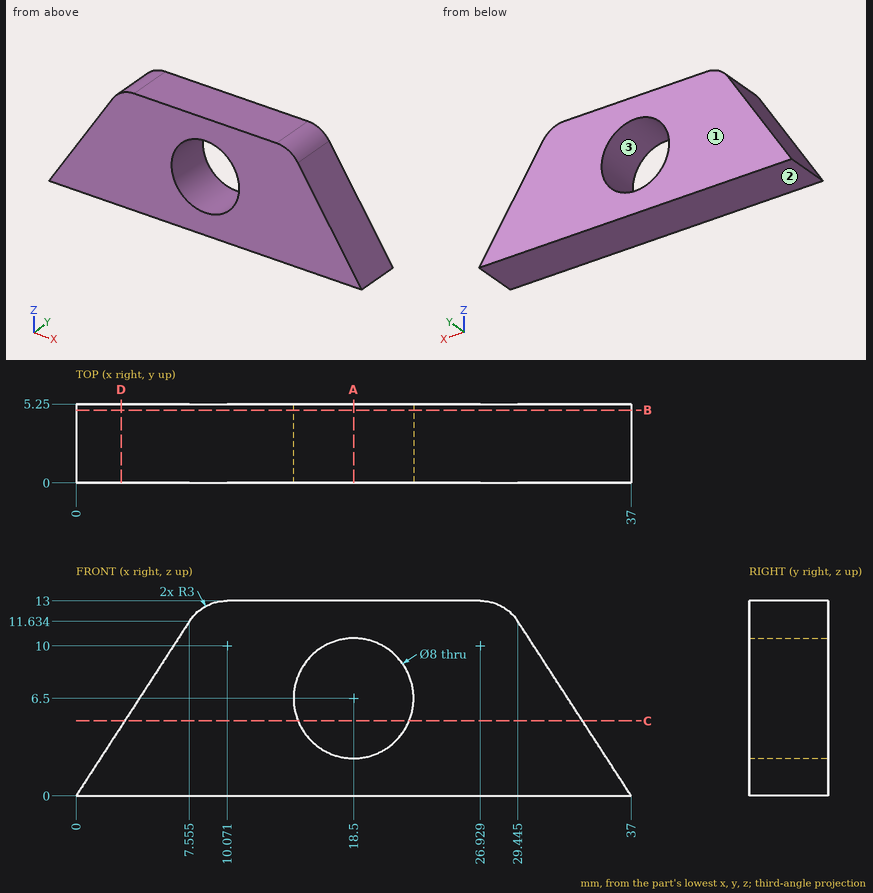
Here's the drawing with two shaded views (mm, measured from the low corner). I have some questions. Give positions to 0.01 mm unless a question says otherwise; leave off trailing zeros. Loops run counter-clockwise (first coordinate to the right, second up) from the corner with the lowest first, then second, coordinate; pieces in that order, holes last. Notation, with made-up numbers: (7, 41.25) -> (41, 41.25) arc R30 cw to (41, 64.25) -> close; hole circle Ø8 at (-16.75, -6.5). An arc over 180 degrees is marked (long way). Answer as a JSON object with one key per item and string values. Group by question number.
Item 1: Imagine slicing it at A-A on x = 18.5. Write out the boundary of the cut face in (y, z).
Item 2: I need wall thicknesses on L1, parallel to Z at x = 18.5, y = 3.05; L2, parallel to X at y = 2.9, z = 8.75; L3, parallel to Z at x = 21.5, y = 0.5 (1 decimal). Which ranges of each line are inside material? Lowest first, please.
Item 3: Will these pins go through, and if not, where does the flat tip stop? pin 1 (1.5 mm diameter, centred on y = 2, z = 4.5, fed in from -X) (1 decimal); pin 2 (3 mm diameter, centred on y = 1, z = 8.5, fed in from -X).
Item 4: Thinking about a two-plate mould opening in Z: for the marked faces 1, 2 and 3, which applies, pulls with the +Z half, pulls with the -Z half, needs draft (parallel to the pull), parting line crosses it, or undercut?
Item 5: Imagine slicing it at D-D on x = 3. Write out the boundary of the cut face in (y, z).
Item 6: Imagine slicing it at C-C on z = 5. Write out the boundary of the cut face in (x, y), then the cut area to 3 significant figures.
Item 7: Imagine slicing it at B-B on y = 4.85. Write out the boundary of the cut face in (x, z) (1 decimal).
Answer list:
{
 "1": {"outline": "(0, 0) -> (5.25, 0) -> (5.25, 2.5) -> (0, 2.5) -> close; (0, 10.5) -> (5.25, 10.5) -> (5.25, 13) -> (0, 13) -> close"},
 "2": {"L1": "z = 0 to 2.5, 10.5 to 13", "L2": "x = 5.68 to 15.19, 21.81 to 31.32", "L3": "z = 0 to 3.9, 9.1 to 13"},
 "3": {"pin 1": "stops at x = 2.4", "pin 2": "stops at x = 4.55"},
 "4": {"face 1": "needs draft", "face 2": "pulls with the -Z half", "face 3": "undercut"},
 "5": {"outline": "(0, 0) -> (5.25, 0) -> (5.25, 4.62) -> (0, 4.62) -> close"},
 "6": {"outline": "(3.25, 0) -> (14.79, 0) -> (14.79, 5.25) -> (3.25, 5.25) -> close; (22.21, 0) -> (33.75, 0) -> (33.75, 5.25) -> (22.21, 5.25) -> close", "area": "121 mm2"},
 "7": {"outline": "(0, 0) -> (37, 0) -> (29.4, 11.6) arc R3 ccw to (26.9, 13) -> (10.1, 13) arc R3 ccw to (7.6, 11.6) -> close; hole circle Ø8 at (18.5, 6.5)"}
}
